Design review of the part shown in the three views and the two pictorial views. Dimensions are in mm from the part's minimum x, y and z. A direction names the side the tool comes from. Give positions to 0.01 mm unless a question says otherwise; leave off trailing zeros. Order: outer loops, then holes, each group sorted by start corner. A loop starts at its lowest first (then second) coordinate and runs counter-clockwise, first axis right, second up. Notation, with made-up numbers: (77.25, 82) -> (125.25, 82) arc R13 cw to (125.25, 87) -> close; hole circle Ø9 at (21.5, 41.5). An arc over 180 degrees is marked (long way). Answer in a Markdown table with one row per item. Add a question column.
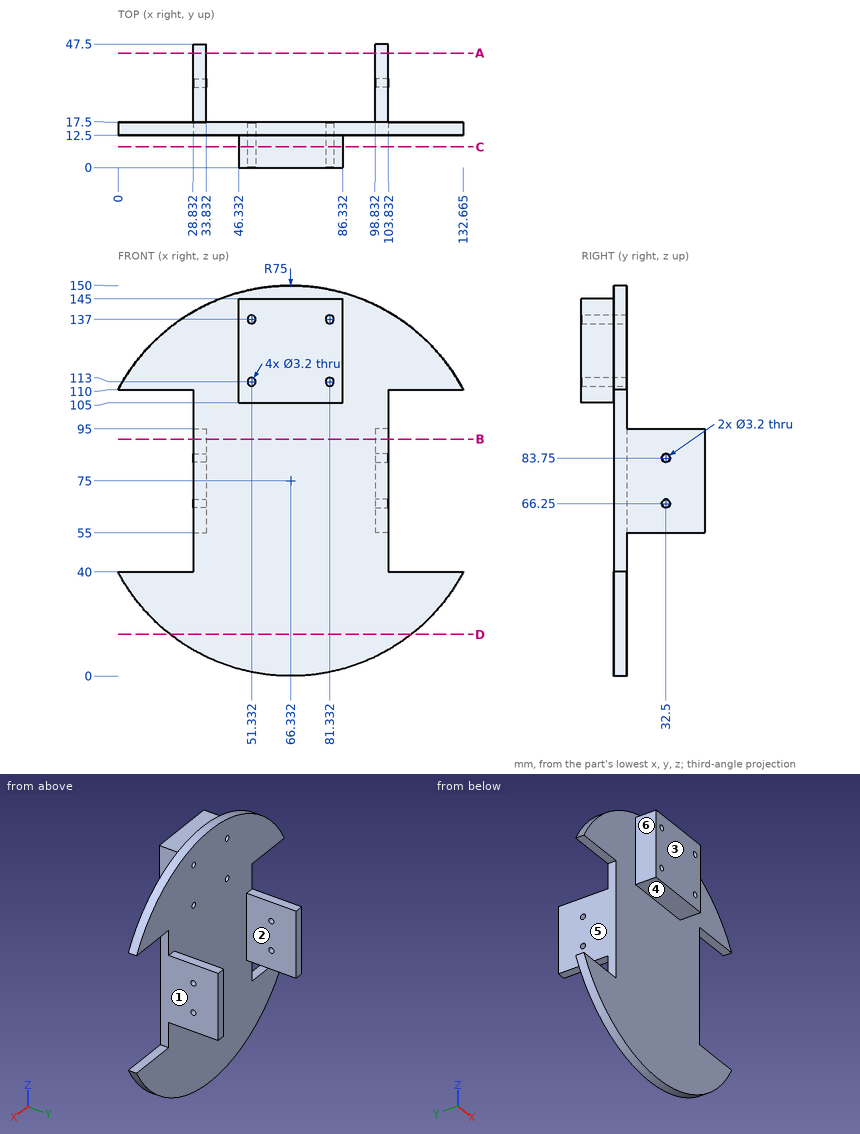
1) Clearance check with flat-ended pins moving along their axes: P1, Ø3.5, axis at x = 51.33, z = 137, coming from the +Y side; P2, Ø14, axis at x = 56.5, y = 7, coming from the -Z side; P3, Ø2.5, axis at x = 101.5, y = 33.5, coming from the -Z side; P4, Ø1, axis at x = 58.5, z = 115, coming from the -Y side. State where each tip first meets the part, or that it passes through.
2) Add section D-D, the plane z = 16. Write out the cut boundary in (x, y) (1 decimal), and give its area (3 significant figures).
3) Add section C-C, the plane y = 8. Write out the cut boundary in (x, z), and give its area (3 significant figures).
4) For L1, parallel to Z at x = 99.9, y = 32.5; L2, parallel to X at y = 6.5, z = 113; L3, parallel to Z at x = 81.5, y = 9.5, list the stretches that pass through material, from the lowest coordinate up.
5) Add section A-A, the plane y = 44. Write out the cut boundary in (x, z).
6) Add section B-B, the plane z = 91. Write out the cut boundary in (x, y).
7) Machinability: for the marked faces 1, 2 and 3, which of the approach directions +Z, -Z, +X, -X, +Y, -Y give a long, thin tool a straight path to every point of the face, cutting with its end or side? Answer none if there is none.
8) Mouldability with a two-part tool opening along Z and no side actions: class the marked faces 4, 5 and 6 as +Z half, -Z half, draft (parallel to the pull), parting line (faces both ways), or undercut.
Verdict:
| question | item | result |
|---|---|---|
| 1 | P1 | stops at y = 17.5 |
| 1 | P2 | stops at z = 0.2 |
| 1 | P3 | stops at z = 55 |
| 1 | P4 | stops at y = 0 |
| 2 | outline | (20, 12.5) -> (112.6, 12.5) -> (112.6, 17.5) -> (20, 17.5) -> close |
| 2 | area | 463 mm2 |
| 3 | outline | (46.33, 105) -> (86.33, 105) -> (86.33, 145) -> (46.33, 145) -> close; hole circle Ø3.2 at (51.33, 113); hole circle Ø3.2 at (51.33, 137); hole circle Ø3.2 at (81.33, 113); hole circle Ø3.2 at (81.33, 137) |
| 3 | area | 1,570 mm2 |
| 4 | L1 | z = 55 to 64.65, 67.85 to 82.15, 85.35 to 95 |
| 4 | L2 | x = 46.33 to 49.73, 52.93 to 79.73, 82.93 to 86.33 |
| 4 | L3 | z = 105 to 111.41, 114.59 to 135.41, 138.59 to 145 |
| 5 | outline | (28.83, 55) -> (33.83, 55) -> (33.83, 95) -> (28.83, 95) -> close; (98.83, 55) -> (103.83, 55) -> (103.83, 95) -> (98.83, 95) -> close |
| 6 | outline | (28.83, 12.5) -> (103.83, 12.5) -> (103.83, 47.5) -> (98.83, 47.5) -> (98.83, 17.5) -> (33.83, 17.5) -> (33.83, 47.5) -> (28.83, 47.5) -> close |
| 7 | face 1 | +X, +Y, -Y |
| 7 | face 2 | +Z, -Z, +Y |
| 7 | face 3 | +Z, -Z, +X, -X, -Y |
| 8 | face 4 | -Z half |
| 8 | face 5 | undercut |
| 8 | face 6 | draft |
